Work out the finished part from the listing and answer in its coordinate system (mm). Face numbers are marked on the shaded views. A direction names the side the tool comes from. Round coordinates to 2 decimals unless told otherwise and drop trailing zeros. Order: outer loops, then holes, each group sorted by start corner. A loop starts at its lowest first (then second) coordinate and runs counter-clockwise, first axis right, second up. Notation, with made-up numbers: (69, 47.5) - (103, 47.5) arc R24 ccw to (103, 81.5) - close; hole circle Ø3 at (-13, 9.5). An arc over 180 degrees is marked (long way). Answer in a Markdown table with one row per item.
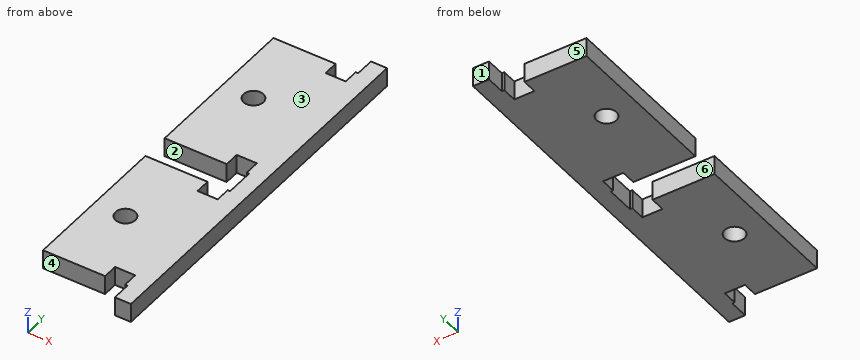
from build123d import *

# Parameters (mm, degrees)
SKETCH2_W               = 40.64
SKETCH2_H               = 127
BOSS_EXTRUDE1_DEPTH     = 6.35
M6_CLEARANCE_HOLE1_D    = 6.6
CUT_EXTRUDE1_DEPTH      = 134.495063954
CUT_EXTRUDE1_DEPTH_BACK = 134.495063954
SKETCH5_W               = 7.0505
SKETCH5_H               = 127
SKETCH6_W               = 25.85012
SKETCH6_H               = 3.175
SKETCH6_W_2             = 27.8745
CUT_EXTRUDE2_DEPTH      = 134.495063954
SKETCH7_W               = 6.35
SKETCH7_H               = 4.7625
CUT_EXTRUDE3_DEPTH      = 134.495063954


with BuildPart() as part:
    # Sketch2 → Boss-Extrude1 (new body)
    with BuildSketch(Plane.XY):
        with Locations((20.32, 63.5)):
            Rectangle(SKETCH2_W, SKETCH2_H)
    extrude(amount=BOSS_EXTRUDE1_DEPTH)

    # M6 Clearance Hole1 (through all)
    with Locations(Plane.XY.offset(6.35)):
        with Locations((17.4625, 31.75), (17.4625, 95.25)):
            Hole(M6_CLEARANCE_HOLE1_D / 2)

    # Sketch5 → Cut-Extrude1 (cut, two sides: drawn at the far end of the back side and taken through both)
    with BuildSketch(Plane.XY.offset(6.35).offset(-CUT_EXTRUDE1_DEPTH_BACK)):
        with Locations((3.52525, 63.5)):
            Rectangle(SKETCH5_W, SKETCH5_H)
    extrude(amount=CUT_EXTRUDE1_DEPTH + CUT_EXTRUDE1_DEPTH_BACK, mode=Mode.SUBTRACT)

    # Sketch6 → Cut-Extrude2 (cut, through all)
    with BuildSketch(Plane.XY.offset(6.35)):
        Polygon((7.0505, 123.825), (7.0505, 120.65), (35.28187, 120.65), (35.28187, 127), (32.90062, 127), (32.90062, 123.825), align=None)
        with Locations((19.97556, 125.4125)):
            Rectangle(SKETCH6_W, SKETCH6_H)
        Polygon((35.28187, 66.675), (7.0505, 66.675), (7.0505, 63.5), (32.90062, 63.5), (32.90062, 60.325), (7.0505, 60.325), (7.0505, 57.15), (35.28187, 57.15), align=None)
        with Locations((19.97556, 61.9125)):
            Rectangle(SKETCH6_W, SKETCH6_H)
        Polygon((35.28187, 0), (35.28187, 6.35), (7.0505, 6.35), (7.0505, 3.175), (34.925, 3.175), (34.925, 0), align=None)
        with Locations((20.98775, 1.5875)):
            Rectangle(SKETCH6_W_2, SKETCH6_H)
    extrude(amount=-CUT_EXTRUDE2_DEPTH, mode=Mode.SUBTRACT)

    # Sketch7 → Cut-Extrude3 (cut, through all)
    with BuildSketch(Plane.XY.offset(6.35)):
        with Locations((31.115, 8.73125)):
            Rectangle(SKETCH7_W, SKETCH7_H)
        Polygon((27.94, 11.1125), (34.29, 11.1125), (34.29, 6.35), (34.4805, 6.35), (34.4805, 11.303), (27.7495, 11.303), (27.7495, 6.35), (27.94, 6.35), align=None)
        Polygon((34.4805, 6.35), (34.29, 6.35), (27.94, 6.35), (27.7495, 6.35), (27.7495, 6.1595), (34.4805, 6.1595), align=None)
        with Locations((31.115, 54.76875)):
            Rectangle(SKETCH7_W, SKETCH7_H)
        Polygon((34.4805, 57.15), (34.29, 57.15), (34.29, 52.3875), (27.94, 52.3875), (27.94, 57.15), (27.7495, 57.15), (27.7495, 52.197), (34.4805, 52.197), align=None)
        Polygon((27.94, 57.15), (34.29, 57.15), (34.4805, 57.15), (34.4805, 57.3405), (27.7495, 57.3405), (27.7495, 57.15), align=None)
        Polygon((34.4805, 66.675), (34.29, 66.675), (27.94, 66.675), (27.7495, 66.675), (27.7495, 66.4845), (34.4805, 66.4845), align=None)
        with Locations((31.115, 69.05625)):
            Rectangle(SKETCH7_W, SKETCH7_H)
        Polygon((27.94, 71.4375), (34.29, 71.4375), (34.29, 66.675), (34.4805, 66.675), (34.4805, 71.628), (27.7495, 71.628), (27.7495, 66.675), (27.94, 66.675), align=None)
        with Locations((31.115, 118.26875)):
            Rectangle(SKETCH7_W, SKETCH7_H)
        Polygon((27.7495, 115.697), (34.4805, 115.697), (34.4805, 120.65), (34.29, 120.65), (34.29, 115.8875), (27.94, 115.8875), (27.94, 120.65), (27.7495, 120.65), align=None)
        Polygon((34.29, 120.65), (34.4805, 120.65), (34.4805, 120.8405), (27.7495, 120.8405), (27.7495, 120.65), (27.94, 120.65), align=None)
    extrude(amount=-CUT_EXTRUDE3_DEPTH, mode=Mode.SUBTRACT)


solid = part.part
1) Find the intervals of material crossed by probe 1 along Y at (x, z) = (33, 1.25); probe 2 along Y at (x, z) = (20, 5.5) (3 decimals); probe 3 along Y at (x, z) = (22, 6.25) (3 decimals), in increasing order. Write a range as from..to.
Filled in:
| item | result |
|---|---|
| probe 1 | y = 11.3..52.2, 71.63..115.7 |
| probe 2 | y = 6.35..29.64, 33.86..57.15, 66.675..93.14, 97.36..120.65 |
| probe 3 | y = 6.35..57.15, 66.675..120.65 |
2) Find section C-C, the plane z = 2.25. Give the number of separate pieces and of enclosed holes in the cut face, then the cut area to 3 significant figures.
Filled in:
| item | result |
|---|---|
| separate pieces | 1 |
| enclosed holes | 2 |
| area | 3,440 mm^2 |
3) Find section D-D, the plane x = 19. Give the vertices of the cut face in (y, z) (3 decimals), then the cut area to 3 significant figures.
Filled in:
| item | result |
|---|---|
| outline | (6.35, 0) - (28.83, 0) - (28.83, 6.35) - (6.35, 6.35) - close; (34.67, 0) - (57.15, 0) - (57.15, 6.35) - (34.67, 6.35) - close; (66.675, 0) - (92.33, 0) - (92.33, 6.35) - (66.675, 6.35) - close; (98.17, 0) - (120.65, 0) - (120.65, 6.35) - (98.17, 6.35) - close |
| area | 591 mm^2 |
4) Which of the six approach directions +Z, -Z, +X, -X, +Y, -Y give full straight-line access (tool end or side, diameter ignored) to the marked faces 4, 5 and 6?
Filled in:
| item | result |
|---|---|
| face 4 | +Z, -Z, -X, -Y |
| face 5 | +Z, -Z, -X, +Y |
| face 6 | +Z, -Z, -X |
5) Find section A-A, the plane y = 117. Give the vertices of the cut face in (x, z), then the cut area to 3 significant figures.
Filled in:
| item | result |
|---|---|
| outline | (7.05, 0) - (27.75, 0) - (27.75, 6.35) - (7.05, 6.35) - close; (34.48, 0) - (40.64, 0) - (40.64, 6.35) - (34.48, 6.35) - close |
| area | 171 mm^2 |
6) Each of these flat-tipped pins is pushed along its axis until it touches: pin 1 (1.9 mm diameter, centred on y = 2, z = 1.5, fed in from -X); pin 2 (1 mm diameter, centred on x = 11.5, z = 2, fed in from +Y); pin 3 (3 mm diameter, centred on x = 12.5, z = 4.5, fed in from -Y); pin 4 (6 mm diameter, centred on x = 17.46, y = 95.25, fed in from +Z). Where does it stop, or does it pass through?
Filled in:
| item | result |
|---|---|
| pin 1 | stops at x = 35.28 |
| pin 2 | stops at y = 120.65 |
| pin 3 | stops at y = 6.35 |
| pin 4 | passes through |
7) Find section B-B, the plane x = 24. Give the vertices of the cut face in (y, z) (3 decimals).
Filled in:
| item | result |
|---|---|
| outline | (6.35, 0) - (57.15, 0) - (57.15, 6.35) - (6.35, 6.35) - close; (66.675, 0) - (120.65, 0) - (120.65, 6.35) - (66.675, 6.35) - close |
8) The mould has two halves that part along Y. Classify the marked faces 1, 2 and 3: released by +Y, released by -Y, zero draft, split by the parting line, or undercut.
Filled in:
| item | result |
|---|---|
| face 1 | released by +Y |
| face 2 | undercut |
| face 3 | zero draft |
